from build123d import *

# Parameters (mm, degrees)
SKETCH2_R               = 2.5
BASE_FLANGE1_DEPTH      = 0.75
EDGE_FLANGE1_DEPTH      = 66.001893912
EDGE_FLANGE1_BEND_DEPTH = 66.001893912
BREAK_CORNER1_START     = -6.85
BREAK_CORNER1_DEPTH     = 13.7


# Read off the part's stored shape, not the designer's step: Break-Corner1
# Sheet-metal steps are written as plain solids
with BuildPart() as part:
    # Sketch2 → Base-Flange1 (new body)
    with BuildSketch(Plane(origin=(0, 0, 0), x_dir=(1, 0, 0), z_dir=(0, 1, 0))):
        with BuildLine():
            Line((-33.000946956, 6), (33.000946956, 6))
            ThreePointArc((33.000946956, 6), (39.000946956, 0), (33.000946956, -6))
            Line((33.000946956, -6), (-33.000946956, -6))
            ThreePointArc((-33.000946956, -6), (-39.000946956, 0), (-33.000946956, 6))
        make_face()
        with Locations(Location((33.000946956, 0, 0), (0, 0, 270))):
            Circle(SKETCH2_R, mode=Mode.SUBTRACT)
        with Locations(Location((-33.000946956, 0, 0), (0, 0, 270))):
            Circle(SKETCH2_R, mode=Mode.SUBTRACT)
    extrude(amount=-BASE_FLANGE1_DEPTH)

    # Edge-Flange1 section (across the edge) → Edge-Flange1 (add)
    with BuildSketch(Plane(origin=(-33.000946956, 0, 6.1), x_dir=(0, 0, -1), z_dir=(1, 0, 0))):
        with BuildLine():
            Line((-0.75, 0.1), (-0.75, 1.25))
            Line((-0.75, 1.25), (0, 1.25))
            Line((0, 1.25), (0, 0.1))
            ThreePointArc((0, 0.1), (0.029289322, 0.029289322), (0.1, 0))
            Line((0.1, 0), (0.1, -0.75))
            ThreePointArc((0.1, -0.75), (-0.501040764, -0.501040764), (-0.75, 0.1))
        make_face()
    extrude(amount=EDGE_FLANGE1_DEPTH)

    # Edge-Flange1 section 2 (across the edge) → Edge-Flange1 bend (add)
    with BuildSketch(Plane(origin=(33.000946956, 0, -6.1), x_dir=(0, 0, 1), z_dir=(-1, 0, 0))):
        with BuildLine():
            Line((-0.75, 0.1), (-0.75, 1.25))
            Line((-0.75, 1.25), (0, 1.25))
            Line((0, 1.25), (0, 0.1))
            ThreePointArc((0, 0.1), (0.029289322, 0.029289322), (0.1, 0))
            Line((0.1, 0), (0.1, -0.75))
            ThreePointArc((0.1, -0.75), (-0.501040764, -0.501040764), (-0.75, 0.1))
        make_face()
    extrude(amount=EDGE_FLANGE1_BEND_DEPTH)

    # Break-Corner1 outline → Break-Corner1 (cut)
    with BuildSketch(Plane.XY.offset(BREAK_CORNER1_START)):
        with BuildLine():
            ThreePointArc((-33.000946956, 0.25), (-32.708053737, 0.957106781), (-32.000946956, 1.25))
            Line((-32.000946956, 1.25), (-33.000946956, 1.25))
            Line((-33.000946956, 1.25), (-33.000946956, 0.25))
        make_face()
        with BuildLine():
            ThreePointArc((32.000946956, 1.25), (32.708053737, 0.957106781), (33.000946956, 0.25))
            Line((33.000946956, 0.25), (33.000946956, 1.25))
            Line((33.000946956, 1.25), (32.000946956, 1.25))
        make_face()
    extrude(amount=BREAK_CORNER1_DEPTH, mode=Mode.SUBTRACT)


solid = part.part
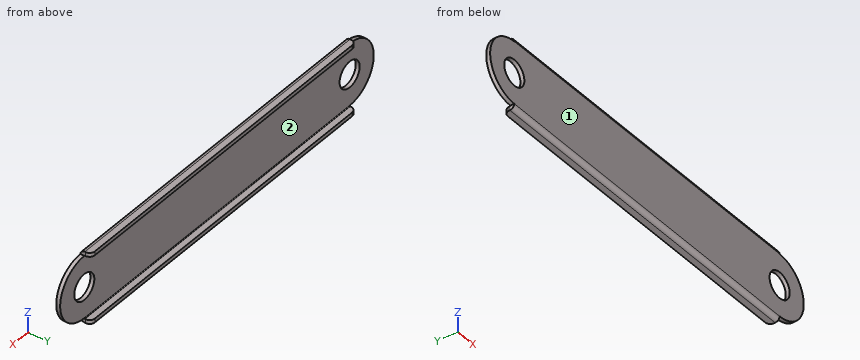
Can you work these out from the model? Positions are in its coordinate system, mm. Face numbers are marked on the shaded views. Coordinates: 2 decimals unless noted, no trailing zeros. Loops run counter-clockwise (first coordinate to the right, second up) from the corner with the lowest first, then second, coordinate; pieces in that order, holes last. Notation, with made-up numbers: M -31,13 L -18,13 A21 ccw -18,47 Z; hole C 12,53.25 d2. An arc over 180 degrees is marked long. Answer as CSV lines item,"result". Start each with the question number.
1. Suppose I cut it at C-C, the plane y = 0.8. List the corners of the cut face in (x, z) for me.
2. For pin 1 Ø6 at (x, z) = (-2.5, -1) entering from +Y; pin 2 Ø6.5 at (x, z) = (-33, 0) entering from -Y; pin 3 Ø0.7 at (y, z) = (0, 6.5) entering from +X, each with a flat end and sliding along its axis, tell me the tip position at first contact or that it passes through.
3. Suppose I cut it at D-D, the plane z = 3.5. List the corners of the cut face in (x, y) for me, plus the area to 3 significant figures.
4. If I drill on probe 1 along X at (y, z) = (-0.35, 0); probe 2 along Z at (x, y) = (0, 0.4); probe 3 along Y at (x, z) = (34.5, 5), over which ranges is the centre line in solid material (lowest first)? Write a range as [from, to].
5. Suppose I cut it at A-A, the plane z = 0. List the corners of the cut face in (x, y) for me.
6. Suppose I cut it at B-B, the plane x = 29. List the corners of the cut face in (y, z) for me.
7. Thinking about a two-plate mould opening in Z: for the marked faces 1 and 2, which applies, +Z half, -Z half, draft (parallel to the pull), parting line (faces both ways), or undercut?
Output:
1,outline,"M -32.84,-6.85 L 32.84,-6.85 L 32.84,-6.1 L -32.84,-6.1 Z; M -32.84,6.1 L 32.84,6.1 L 32.84,6.85 L -32.84,6.85 Z"
2,pin 1,"stops at y = 0"
2,pin 2,"stops at y = -0.75"
2,pin 3,"stops at x = 33"
3,outline,"M -37.87,-0.75 L 37.87,-0.75 L 37.87,0 L -37.87,0 Z"
3,area,"56.8 mm^2"
4,probe 1,"x = [-39, -35.5], [-30.5, 30.5], [35.5, 39]"
4,probe 2,"z = [-6.85, -6.1], [6.1, 6.85]"
4,probe 3,"y = [-0.75, 0]"
5,outline,"M -39,-0.75 L -35.5,-0.75 L -35.5,0 L -39,0 Z; M -30.5,-0.75 L 30.5,-0.75 L 30.5,0 L -30.5,0 Z; M 35.5,-0.75 L 39,-0.75 L 39,0 L 35.5,0 Z"
6,outline,"M -0.75,-6 A0.85 ccw 0.1,-6.85 L 1.25,-6.85 L 1.25,-6.1 L 0.1,-6.1 A0.1 cw 0,-6 L 0,6 A0.1 cw 0.1,6.1 L 1.25,6.1 L 1.25,6.85 L 0.1,6.85 A0.85 ccw -0.75,6 Z"
7,face 1,"draft"
7,face 2,"undercut"
